Answer from the drawing. Dimensions are ordinates in mm from the lowest x, y and z of the part. A direction names the side the tool comes from. Give positions to 0.01 mm unless a question says otherwise; leave off trailing zeros. Loops run counter-clockwise (first coordinate to the right, second up) from the corner with the lowest first, then second, coordinate; pieces in that order, holes last. Notation, with made-up numbers: M 67.25,77 L 88.25,77 A5 ccw 88.25,83 Z; hole C 32,61 d3. An arc over 180 degrees is marked long. Use a Markdown table: item, result.
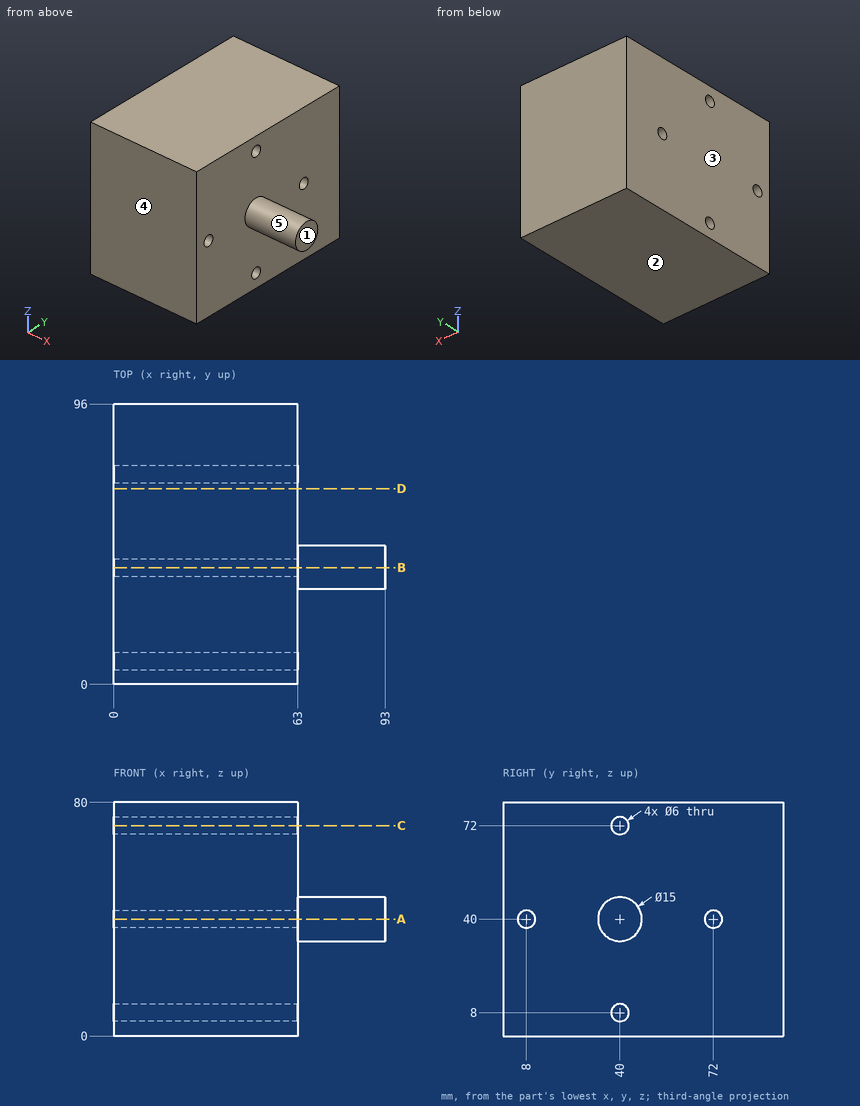
(1) A cutting plane is placed at A-A (z = 40). Write down the section's boundary in (x, y), and give its area (3 significant figures).
Entries:
| item | result |
|---|---|
| outline | M 0,0 L 63,0 L 63,5 L 0,5 Z; M 0,11 L 63,11 L 63,32.5 L 93,32.5 L 93,47.5 L 63,47.5 L 63,69 L 0,69 Z; M 0,75 L 63,75 L 63,96 L 0,96 Z |
| area | 5,740 mm² |
(2) The mould has two halves that part along X. Classify the marked faces 1, 2 and 3: released by +X, released by -X, zero draft, split by the parting line, or undercut.
Entries:
| item | result |
|---|---|
| face 1 | released by +X |
| face 2 | zero draft |
| face 3 | released by -X |
(3) A cutting plane is placed at D-D (y = 67). Write down the section's boundary in (x, z).
Entries:
| item | result |
|---|---|
| outline | M 0,0 L 63,0 L 63,80 L 0,80 Z |
(4) A cutting plane is placed at C-C (z = 72). Write down the section's boundary in (x, y), and give its area (3 significant figures).
Entries:
| item | result |
|---|---|
| outline | M 0,0 L 63,0 L 63,37 L 0,37 Z; M 0,43 L 63,43 L 63,96 L 0,96 Z |
| area | 5,670 mm² |
(5) Which of the six approach directions +Z, -Z, +X, -X, +Y, -Y give full straight-line access (tool end or side, diameter ignored) to the marked faces 4 and 5?
Entries:
| item | result |
|---|---|
| face 4 | +Z, -Z, +X, -X, -Y |
| face 5 | +X |
(6) A cutting plane is placed at B-B (y = 40). Write down the section's boundary in (x, z).
Entries:
| item | result |
|---|---|
| outline | M 0,0 L 63,0 L 63,5 L 0,5 Z; M 0,11 L 63,11 L 63,32.5 L 93,32.5 L 93,47.5 L 63,47.5 L 63,69 L 0,69 Z; M 0,75 L 63,75 L 63,80 L 0,80 Z |
(7) Given P1, Ø6, axis at y = 55.5, z = 32, coming from the +X side, flat-ended and moving along its own axis, determine where the tip first touches the part or whether it passes through.
Entries:
| item | result |
|---|---|
| P1 | stops at x = 63 |
(8) Consider probe 1 along Z at (x, y) = (38, 39); probe 2 along Y at (x, z) = (46, 8); probe 3 along X at (y, z) = (33, 5.5). Determine where each line is inside the solid, lowest interval first. Write a range as [from, to].
Entries:
| item | result |
|---|---|
| probe 1 | z = [0, 5.17], [10.83, 69.17], [74.83, 80] |
| probe 2 | y = [0, 37], [43, 96] |
| probe 3 | x = [0, 63] |
